Verification items for this drawing (mm, ordinates from the low corner). A direction names the side the tool comes from. Round coordinates to 2 decimals unless told otherwise and drop trailing zeros. Loops run counter-clockwise (first coordinate to the right, second up) from the corner with the lowest first, then second, coordinate; pieces in that order, holes last. Notation, with made-up numbers: M 10.25,15.25 L 51.25,15.25 A17 cw 51.25,31.25 Z; hole C -26,71.5 d11. An arc over 180 degrees is marked long. Write item = value, one per line. Start each with the question number.
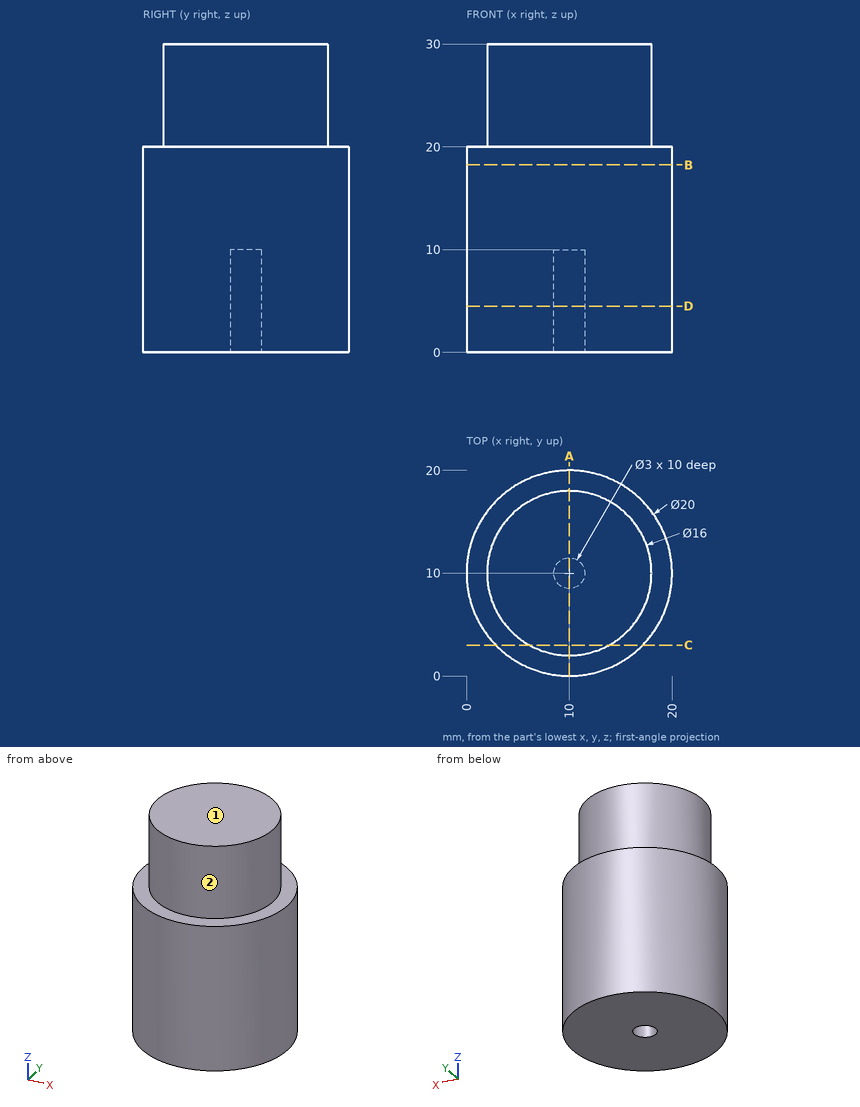
1. Tool access check on the marked faces 1 and 2. Record the directions out of +Z, -Z, +X, -X, +Y, -Y that give a thin tool (end or side, any length) a straight path to the whole face; none if there is none.
2. Section check B-B, the plane z = 18.25. Enter the section's corners in (x, y), and give its area (3 significant figures).
3. Section check C-C, the plane y = 3. Enter the section's corners in (x, z), and give its area (3 significant figures).
4. Section check A-A, the plane x = 10. Enter the section's corners in (y, z), and give its area (3 significant figures).
5. Gauge pin test, flat ends, axial feed: P1, Ø2, axis at y = 7.5, z = 14, coming from the -X side; P2, Ø3, axis at y = 6, z = 17, coming from the +X side; P3, Ø3, axis at x = 7, z = 15.5, coming from the +Y side. Record the tip position at first contact, or that the pin passes through.
6. Section check D-D, the plane z = 4.5. Enter the section's corners in (x, y), and give its area (3 significant figures).
7. Thickness scan on line 1 (Y direction, x = 10, z = 4.5); line 2 (Z direction, x = 2.25, y = 14.25); line 3 (Y direction, x = 14, z = 7.5). Record the ranges inside material, lowest first.
Computed values:
q1.face_1 = +Z, +X, -X, +Y, -Y
q1.face_2 = +Z
q2.outline = C 10,10 d20
q2.area = 314 mm2
q3.outline = M 2.86,0 L 17.14,0 L 17.14,20 L 13.87,20 L 13.87,30 L 6.13,30 L 6.13,20 L 2.86,20 Z
q3.area = 363 mm2
q4.outline = M 0,0 L 8.5,0 L 8.5,10 L 11.5,10 L 11.5,0 L 20,0 L 20,20 L 18,20 L 18,30 L 2,30 L 2,20 L 0,20 Z
q4.area = 530 mm2
q5.P1 = 0.11
q5.P2 = 19.68
q5.P3 = 19.89
q6.outline = C 10,10 d20; hole C 10,10 d3
q6.area = 307 mm2
q7.line_1 = 0 to 8.5, 11.5 to 20
q7.line_2 = 0 to 20
q7.line_3 = 0.83 to 19.17
